```python
from build123d import *

# Parameters (mm, degrees)
F1_DEPTH = 60


with BuildPart() as f1:
    # F0 (on Top) → F1 (new body)
    with BuildSketch(Plane.XY):
        with BuildLine():
            ThreePointArc((-306, 6), (-304.242641, 1.757359), (-300, 0))
            Line((-300, 0), (-246, 0))
            ThreePointArc((-246, 0), (-241.757359, 1.757359), (-240, 6))
            Line((-240, 6), (-240, 21))
            Line((-240, 21), (-244, 21))
            Line((-244, 21), (-244, 6))
            ThreePointArc((-244, 6), (-244.585786, 4.585786), (-246, 4))
            Line((-246, 4), (-300, 4))
            ThreePointArc((-300, 4), (-301.414214, 4.585786), (-302, 6))
            Line((-302, 6), (-302, 431))
            ThreePointArc((-302, 431), (-301.414214, 432.414214), (-300, 433))
            Line((-300, 433), (300, 433))
            ThreePointArc((300, 433), (301.414214, 432.414214), (302, 431))
            Line((302, 431), (302, 6))
            ThreePointArc((302, 6), (301.414214, 4.585786), (300, 4))
            Line((300, 4), (246, 4))
            ThreePointArc((246, 4), (244.585786, 4.585786), (244, 6))
            Line((244, 6), (244, 21))
            Line((244, 21), (240, 21))
            Line((240, 21), (240, 6))
            ThreePointArc((240, 6), (241.757359, 1.757359), (246, 0))
            Line((246, 0), (300, 0))
            ThreePointArc((300, 0), (304.242641, 1.757359), (306, 6))
            Line((306, 6), (306, 431))
            ThreePointArc((306, 431), (304.242641, 435.242641), (300, 437))
            Line((300, 437), (-300, 437))
            ThreePointArc((-300, 437), (-304.242641, 435.242641), (-306, 431))
            Line((-306, 431), (-306, 6))
        make_face()
    extrude(amount=-F1_DEPTH)


solid = f1.part
```
Geometry check sheet. Reference: the model listing, model coordinates, mm. A direction names the side the tool comes from. Coordinates: 2 decimals unless noted, no trailing zeros. Order: outer loops, then holes, each group sorted by start corner. A loop starts at its lowest first (then second) coordinate and runs counter-clockwise, first axis right, second up.
Q1. Sectioned sample at B-B on z = -38. Record the cut outline in (x, y).
Reply:
outline: (-306, 6) arc R6 ccw to (-300, 0) - (-246, 0) arc R6 ccw to (-240, 6) - (-240, 21) - (-244, 21) - (-244, 6) arc R2 cw to (-246, 4) - (-300, 4) arc R2 cw to (-302, 6) - (-302, 431) arc R2 cw to (-300, 433) - (300, 433) arc R2 cw to (302, 431) - (302, 6) arc R2 cw to (300, 4) - (246, 4) arc R2 cw to (244, 6) - (244, 21) - (240, 21) - (240, 6) arc R6 ccw to (246, 0) - (300, 0) arc R6 ccw to (306, 6) - (306, 431) arc R6 ccw to (300, 437) - (-300, 437) arc R6 ccw to (-306, 431) - close
Q2. Draft check along X on faces 1 (the face through (-273, 4, -30)), 2 (the face through (306, 216, -30)), 3 (the face through (-306, 221, -30)), 4 (the face through (-273, 0, -30)). Enter one of: released by +X, released by -X, zero draft, split by the parting line, or undercut.
Reply:
face 1: undercut
face 2: released by +X
face 3: released by -X
face 4: zero draft
Q3. Thickness scan on probe 1 along X at (y, z) = (28.5, -36); probe 2 along Y at (x, z) = (89, -42.5). Record the ranges inside material, lowest first.
Reply:
probe 1: x = -306 to -302, 302 to 306
probe 2: y = 433 to 437
Q4. Depth check by flat-ended pin: pin 1 Ø1 at (x, z) = (-204, -27.5) entering from -Y. Enter the tip coordinate at first touch or a pass-through.
Reply:
pin 1: stops at y = 433
Q5. Tool access check on faces 5 (the face through (-240, 13, -30)), 6 (the face through (244, 13, -30)), 7 (the face through (273, 0, -30)). Record the directions out of +Z, -Z, +X, -X, +Y, -Y that give a thin tool (end or side, any length) a straight path to the whole face; none if there is none.
Reply:
face 5: +Z, -Z, -Y
face 6: +Z, -Z
face 7: +Z, -Z, +X, -X, -Y
Q6. Sectioned sample at A-A on y = 139.5. Record the cut outline in (x, z).
Reply:
outline: (-306, -60) - (-302, -60) - (-302, 0) - (-306, 0) - close; (302, -60) - (306, -60) - (306, 0) - (302, 0) - close
Q7. Sectioned sample at C-C on x = 69. Record the cut outline in (y, z).
Reply:
outline: (433, -60) - (437, -60) - (437, 0) - (433, 0) - close
